Input: part model. Units: mm. Frame: model coordinates. Round coordinates to 2 decimals unless told otherwise and drop trailing zeros. Order: outer loops, then holes, each group sorted by start corner. A loop starts at its lowest first (then second) coordinate and runs counter-clockwise, first axis right, second up. Notation, with made-up numbers: (-5.75, -18.5) -> (39.25, -18.5) arc R8 ccw to (39.25, -8.5) -> close; hole circle Ø9 at (-9.5, 35). An arc over 180 degrees is marked (long way). Answer as CSV lines item,"result". Start each with the question number.
1) First-contact query: P1, Ø9.5, axis at x = 107.95, z = 38.1, coming from the -Y side. Flat tip, straight axial feed; report the tip coordinate or a pass-through.
2) Line query: L1, parallel to X at y = 8.5, z = 1193.8; L2, parallel to Z at x = 35.5, y = 6; L3, parallel to X at y = 13.25, z = 38.1. Output: solid intervals per line, ascending.
3) Mould query, pull axis Z, two halves, no side actions, for faces 1 (the face through (119, 13, 1651)), 2 (the face through (119, 13, 0)), 3 (the face through (26.048, 12.522, 1399.015)), 4 (the face through (0, 13, 837)). Classes: +Z half, -Z half, draft (parallel to the pull), parting line (faces both ways), or undercut.
4) Section query A-A, the plane x = 25.4. Output: boundary loops of the cut face in (y, z), and give its area (3 significant figures).
5) Section query B-B, the plane z = 1193.8. Output: boundary loops of the cut face in (x, y), and give its area (3 significant figures).
```python
from build123d import *

# Parameters (mm, degrees)
SKETCH1_W               = 241.3
SKETCH1_H               = 1651
BOSS_EXTRUDE1_DEPTH     = 25.4
CUT_EXTRUDE1_DEPTH      = 1669.733606661
CUT_EXTRUDE1_DEPTH_BACK = 1669.733606661
SKETCH2_R               = 7.9375
SKETCH3_R               = 14.72946
CUT_EXTRUDE2_DEPTH      = 1669.733606661


with BuildPart() as part:
    # Sketch1 → Boss-Extrude1 (new body)
    with BuildSketch(Plane(origin=(0, 0, 0), x_dir=(1, 0, 0), z_dir=(0, 1, 0))):
        with Locations((120.65, -825.5)):
            Rectangle(SKETCH1_W, SKETCH1_H)
    extrude(amount=BOSS_EXTRUDE1_DEPTH)

    # Sketch2 → Cut-Extrude1 (cut, two sides: drawn at the far end of the back side and taken through both)
    with BuildSketch(Plane(origin=(0, 25.4, 0), x_dir=(1, 0, 0), z_dir=(0, 1, 0)).offset(-CUT_EXTRUDE1_DEPTH_BACK)):
        with Locations(Location((107.95, -38.1, 0), (0, 0, 270))):
            Circle(SKETCH2_R)
        with Locations(Location((107.95, -1449.0573, 0), (0, 0, 270))):
            Circle(SKETCH2_R)
    extrude(amount=CUT_EXTRUDE1_DEPTH + CUT_EXTRUDE1_DEPTH_BACK, mode=Mode.SUBTRACT)

    # Sketch3 → Cut-Extrude2 (cut, through all)
    with BuildSketch(Plane.XZ):
        with Locations(Location((215.9, 1193.8, 0), (0, 0, 270))):
            Circle(SKETCH3_R)
        with Locations(Location((25.4, 1193.8, 0), (0, 0, 270))):
            Circle(SKETCH3_R)
        with Locations(Location((25.4, 1384.3, 0), (0, 0, 270))):
            Circle(SKETCH3_R)
        with Locations(Location((215.9, 1384.3, 0), (0, 0, 270))):
            Circle(SKETCH3_R)
    extrude(amount=-CUT_EXTRUDE2_DEPTH, mode=Mode.SUBTRACT)


solid = part.part
```
Findings:
1,P1,"passes through"
2,L1,"x = 0 to 10.67, 40.13 to 201.17, 230.63 to 241.3"
2,L2,"z = 0 to 1183.08, 1204.52 to 1373.58, 1395.02 to 1651"
2,L3,"x = 0 to 100.01, 115.89 to 241.3"
3,face 1,"+Z half"
3,face 2,"-Z half"
3,face 3,"undercut"
3,face 4,"draft"
4,outline,"(0, 0) -> (25.4, 0) -> (25.4, 1179.07) -> (0, 1179.07) -> close; (0, 1208.53) -> (25.4, 1208.53) -> (25.4, 1369.57) -> (0, 1369.57) -> close; (0, 1399.03) -> (25.4, 1399.03) -> (25.4, 1651) -> (0, 1651) -> close"
4,area,"40,400 mm^2"
5,outline,"(0, 0) -> (10.67, 0) -> (10.67, 25.4) -> (0, 25.4) -> close; (40.13, 0) -> (201.17, 0) -> (201.17, 25.4) -> (40.13, 25.4) -> close; (230.63, 0) -> (241.3, 0) -> (241.3, 25.4) -> (230.63, 25.4) -> close"
5,area,"4,630 mm^2"
